Input: part model. Units: mm. Frame: model coordinates. Face numbers are marked on the shaded views. A direction names the side the tool comes from. Coordinates: 2 decimals unless noted, no trailing zeros. Loops run counter-clockwise (first coordinate to the right, second up) from the corner with the lowest first, then second, coordinate; pieces in that order, holes last. Notation, with made-up numbers: (84.5, 87) - (99.5, 87) arc R12 ccw to (99.5, 100) - close; hole circle Ø9 at (-23.75, -35). An arc over 180 degrees is marked (long way). Use one line per item in the form item = value.
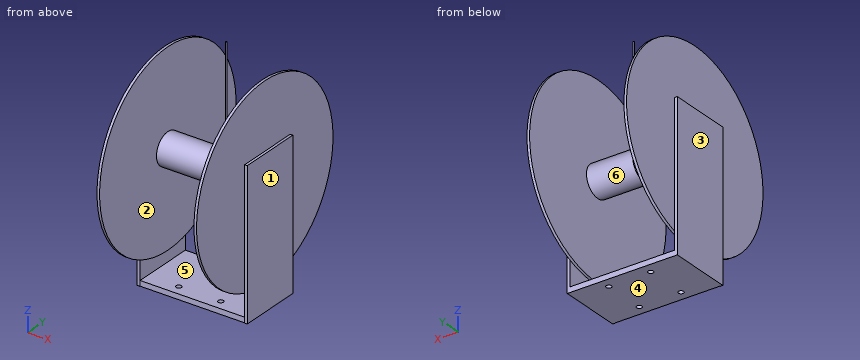
from build123d import *

# Parameters (mm, degrees)
SKETCH1_R           = 228.6
BOSS_EXTRUDE1_DEPTH = 6.35
SKETCH2_R           = 38.1
BOSS_EXTRUDE2_DEPTH = 228.6
SKETCH3_R           = 228.6
BOSS_EXTRUDE3_DEPTH = 6.35
SKETCH4_R           = 38.1
BOSS_EXTRUDE4_DEPTH = 6.35
SKETCH5_R           = 38.1
BOSS_EXTRUDE5_DEPTH = 6.35
BOSS_EXTRUDE6_DEPTH = 6.35
SKETCH7_W           = 203.2
SKETCH7_H           = 152.4
BOSS_EXTRUDE7_DEPTH = 6.35
BOSS_EXTRUDE8_DEPTH = 6.35
SKETCH9_W           = 12.7
SKETCH9_H           = 151.635108104
BOSS_EXTRUDE9_DEPTH = 254
SKETCH10_R          = 6.35
CUT_EXTRUDE1_DEPTH  = 12.7
SKETCH13_R          = 1.59


with BuildPart() as part:
    # Sketch1 → Boss-Extrude1 (new body)
    with BuildSketch(Plane(origin=(0, 0, 0), x_dir=(0, 0, -1), z_dir=(1, 0, 0))):
        Circle(SKETCH1_R)
    extrude(amount=BOSS_EXTRUDE1_DEPTH)

    # Sketch2 → Boss-Extrude2 (add)
    with BuildSketch(Plane(origin=(6.35, 0, 0), x_dir=(0, 0, -1), z_dir=(1, 0, 0))):
        Circle(SKETCH2_R)
    extrude(amount=BOSS_EXTRUDE2_DEPTH)

    # Sketch3 → Boss-Extrude3 (add)
    with BuildSketch(Plane(origin=(234.95, 0, 0), x_dir=(0, 0, -1), z_dir=(1, 0, 0))):
        Circle(SKETCH3_R)
    extrude(amount=BOSS_EXTRUDE3_DEPTH)

    # Sketch4 → Boss-Extrude4 (add)
    with BuildSketch(Plane(origin=(241.3, 0, 0), x_dir=(0, 0, -1), z_dir=(1, 0, 0))):
        Circle(SKETCH4_R)
    extrude(amount=BOSS_EXTRUDE4_DEPTH)

    # Sketch5 → Boss-Extrude5 (add)
    with BuildSketch(Plane.ZY):
        Circle(SKETCH5_R)
    extrude(amount=BOSS_EXTRUDE5_DEPTH)

    # Sketch6 → Boss-Extrude6 (add)
    with BuildSketch(Plane(origin=(247.65, 0, 0), x_dir=(0, 0, -1), z_dir=(1, 0, 0))):
        Polygon((-76.2, -76.2), (-76.2, 0), (-76.2, 76.2), (-5.028509112, 76.2), (76.2, 76.2), (76.2, -76.2), align=None)
    extrude(amount=BOSS_EXTRUDE6_DEPTH)

    # Sketch7 → Boss-Extrude7 (add)
    with BuildSketch(Plane(origin=(254, 0, 0), x_dir=(0, 0, -1), z_dir=(1, 0, 0))):
        with Locations((177.8, 0)):
            Rectangle(SKETCH7_W, SKETCH7_H)
    extrude(amount=-BOSS_EXTRUDE7_DEPTH)

    # Sketch8 → Boss-Extrude8 (add)
    with BuildSketch(Plane.ZY.offset(6.35)):
        Polygon((-76.2, -76.2), (76.2, -76.2), (76.2, 76.2), (-76.2, 76.2), (-279.4, 76.2), (-279.4, -76.2), align=None)
    extrude(amount=BOSS_EXTRUDE8_DEPTH)

    # Sketch9 → Boss-Extrude9 (add)
    with BuildSketch(Plane.ZY.offset(-247.65)):
        with Locations((-273.05, 0.382445948)):
            Rectangle(SKETCH9_W, SKETCH9_H)
    extrude(amount=BOSS_EXTRUDE9_DEPTH)

    # Sketch10 → Cut-Extrude1 (cut)
    with BuildSketch(Plane(origin=(0, 0, -279.4), x_dir=(-1, 0, 0), z_dir=(0, 0, -1))):
        with Locations((-171.45, 50.8)):
            Circle(SKETCH10_R)
        with Locations((-69.85, 50.8)):
            Circle(SKETCH10_R)
        with Locations((-69.85, -50.8)):
            Circle(SKETCH10_R)
        with Locations((-171.45, -50.8)):
            Circle(SKETCH10_R)
    extrude(amount=-CUT_EXTRUDE1_DEPTH, mode=Mode.SUBTRACT)

    # Sweep1: sweep along a path in Sketch12
    with BuildLine(Plane.ZY.offset(-120.65)) as sweep1_path:
        Line((260, 38.1), (0, 38.1))
        ThreePointArc((0, 38.1), (-26.940768363, 26.940768363), (-38.1, 0))
    # Sketch13 → Sweep1 (sweep)
    with BuildSketch(Plane(origin=(0, 0, 0), x_dir=(1, 0, 0), z_dir=(0, 1, 0))):
        with Locations((120.65, 38.1)):
            Circle(SKETCH13_R)
    sweep(path=sweep1_path.line)


solid = part.part
Q1. Cut plane B-B, the plane z = -145.5. Return loops of the section in (x, y).
Check values:
outline = (-12.7, -76.2) - (-6.35, -76.2) - (-6.35, 76.2) - (-12.7, 76.2) - close; (0, -176.32) - (6.35, -176.32) - (6.35, 176.32) - (0, 176.32) - close; (234.95, -176.32) - (241.3, -176.32) - (241.3, 176.32) - (234.95, 176.32) - close; (247.65, -76.2) - (254, -76.2) - (254, 76.2) - (247.65, 76.2) - close
Q2. First-contact query: P1, Ø6, axis at x = 68.5, y = 46.5, coming from the +Z side; P2, Ø4, axis at y = 6, z = 182, coming from the -X side; P3, Ø3, axis at x = 251.5, y = 21, coming from the +Z side. Flat tips, straight axial feed; report the tip coordinate or a pass-through.
Check values:
P1 = -266.7
P2 = 0
P3 = 76.2
Q3. Set-up query: the marked faces 4, 5 and 6. Return all of +Z, -Z, +X, -X, +Y, -Y with unobstructed straight access to the full face (end or side cutting, diameter ignored); none if empty.
Check values:
face_4 = -Z, +X, -X, +Y, -Y
face_5 = +Y, -Y
face_6 = none
Q4. Pull-direction query (X, two-part tool) for the marked faces 1, 2 and 3; classes: pulls with the +X half, pulls with the -X half, needs draft (parallel to the pull), parting line crosses it, or undercut.
Check values:
face_1 = pulls with the +X half
face_2 = undercut
face_3 = pulls with the -X half
Q5. Cut plane C-C, the plane x = 171.45. Return loops of the section in (y, z).
Check values:
outline = (-75.44, -279.4) - (-57.15, -279.4) - (-57.15, -266.7) - (-75.44, -266.7) - close; (-44.45, -279.4) - (44.45, -279.4) - (44.45, -266.7) - (-44.45, -266.7) - close; circle Ø76.2 at (0, 0); (57.15, -279.4) - (76.2, -279.4) - (76.2, -266.7) - (57.15, -266.7) - close
Q6. Ray query, line 1 along Y through (x, z) = (171.45, -272.5); line 2 along X through (y, z) = (29, -112); line 3 along Z through (x, y) = (50, 1.5). Return the intervals inside material, ascending. Write a range as [from, to].
Check values:
line_1 = [-75.44, -57.15], [-44.45, 44.45], [57.15, 76.2]
line_2 = [-12.7, -6.35], [0, 6.35], [234.95, 241.3], [247.65, 254]
line_3 = [-279.4, -266.7], [-38.07, 38.07]
Q7. Cut plane A-A, the plane y = -50.8. Return loops of the section in (x, z).
Check values:
outline = (-12.7, -279.4) - (63.5, -279.4) - (63.5, -266.7) - (-6.35, -266.7) - (-6.35, 76.2) - (-12.7, 76.2) - close; (0, -222.88) - (6.35, -222.88) - (6.35, 222.88) - (0, 222.88) - close; (76.2, -279.4) - (165.1, -279.4) - (165.1, -266.7) - (76.2, -266.7) - close; (177.8, -279.4) - (254, -279.4) - (254, 76.2) - (247.65, 76.2) - (247.65, -266.7) - (177.8, -266.7) - close; (234.95, -222.88) - (241.3, -222.88) - (241.3, 222.88) - (234.95, 222.88) - close
Q8. Cut plane D-D, the plane z = 133.5. Return loops of the section in (x, y), then the cut area to 3 significant figures.
Check values:
outline = (0, -185.57) - (6.35, -185.57) - (6.35, 185.57) - (0, 185.57) - close; circle Ø3.18 at (120.65, 38.1); (234.95, -185.57) - (241.3, -185.57) - (241.3, 185.57) - (234.95, 185.57) - close
area = 4,720 mm²
